from build123d import *

# Parameters (mm, degrees)
SKETCH046_R     = 1.5
PAD026_DEPTH    = 32
POCKET016_DEPTH = 21
SKETCH049_W     = 38.6999153105
SKETCH049_H     = 8
POCKET017_DEPTH = 50
PAD027_DEPTH    = 3
SKETCH050_W     = 42.8952211791
SKETCH050_H     = 8
POCKET018_DEPTH = 32
SKETCH051_R     = 23.5
PAD028_DEPTH    = 1


with BuildPart() as part:
    # Sketch046 → Pad026 (new body)
    with BuildSketch(Plane.XY):
        with BuildLine():
            Line((-21.3218441303, 2.7620577266), (-17, 2))
            Line((-17, 2), (-17, 1))
            Line((-17, 1), (-19, 1))
            Line((-19, 1), (-19, -1))
            Line((-19, -1), (-17, -1))
            Line((-17, -1), (-17, -2))
            Line((-19.3499576553, -2.4143609381), (-17, -2))
            ThreePointArc((-19.3499576553, -2.4143609381), (-18.5993421546, -5.8578555305), (-17.2411687539, -9.11))
            Line((17.2411687539, -9.11), (-17.2411687539, -9.11))
            ThreePointArc((17.2411687539, -9.11), (18.5993421546, -5.8578555305), (19.3499576553, -2.4143609381))
            Line((19.3499576553, -2.4143609381), (17, -2))
            Line((17, -2), (17, -1))
            Line((17, -1), (19, -1))
            Line((19, -1), (19, 1))
            Line((19, 1), (17, 1))
            Line((17, 1), (17, 2))
            Line((17, 2), (21.3218441303, 2.7620577266))
            ThreePointArc((13, -17.1245437895), (19.8334685845, -8.2996098649), (21.3218441303, 2.7620577266))
            Line((13, -17.1245437895), (10, -17.1245437895))
            Line((10, -17.1245437895), (10, -10.1245437895))
            Line((10, -10.1245437895), (-10, -10.1245437895))
            Line((-10, -10.1245437895), (-10, -17.1245437895))
            Line((-10, -17.1245437895), (-13, -17.1245437895))
            ThreePointArc((-21.3218441303, 2.7620577266), (-19.8334685845, -8.2996098649), (-13, -17.1245437895))
        make_face()
        with Locations((-12.5, -15)):
            Circle(SKETCH046_R, mode=Mode.SUBTRACT)
        with Locations((12.5, -15)):
            Circle(SKETCH046_R, mode=Mode.SUBTRACT)
    extrude(amount=PAD026_DEPTH)

    # Sketch047 (on Face28 of Pad026) → Pocket016 (cut)
    with BuildSketch(Plane.XY.offset(32)):
        with BuildLine():
            ThreePointArc((-18.9669083684, -10.1245437895), (-16.3621761284, -13.9473722379), (-13, -17.1245437895))
            Line((-13, -17.1245437895), (13, -17.1245437895))
            ThreePointArc((13, -17.1245437895), (16.3621761284, -13.9473722379), (18.9669083684, -10.1245437895))
            Line((-18.9669083684, -10.1245437895), (18.9669083684, -10.1245437895))
        make_face()
    extrude(amount=-POCKET016_DEPTH, mode=Mode.SUBTRACT)

    # Sketch049 (on Face5 of Pocket016) → Pocket017 (cut)
    with BuildSketch(Plane.XY.offset(32)):
        with Locations((0, 1.5856390619)):
            Rectangle(SKETCH049_W, SKETCH049_H)
    extrude(amount=-POCKET017_DEPTH, mode=Mode.SUBTRACT)

    # Sketch048 (on Face5 of Pocket016) → Pad027 (join)
    with BuildSketch(Plane.XY.offset(32)):
        with BuildLine():
            ThreePointArc((-21.4476105895, 1.5), (-21.02655084, -4.4871104034), (-18.9669083684, -10.1245437895))
            Line((-13, -10.1245437895), (-18.9669083684, -10.1245437895))
            Line((-6, -17.1245437895), (-13, -10.1245437895))
            Line((6, -17.1245437895), (-6, -17.1245437895))
            Line((6, -17.1245437895), (13, -10.1245437895))
            Line((13, -10.1245437895), (18.9669083684, -10.1245437895))
            ThreePointArc((18.9669083684, -10.1245437895), (21.02655084, -4.4871104034), (21.4476105895, 1.5))
            Line((-21.4476105895, 1.5), (21.4476105895, 1.5))
        make_face()
    extrude(amount=PAD027_DEPTH)

    # Sketch050 (on Face24 of Pad027) → Pocket018 (cut)
    with BuildSketch(Plane.XY.offset(32)):
        with Locations((0, 5.5)):
            Rectangle(SKETCH050_W, SKETCH050_H)
    extrude(amount=-POCKET018_DEPTH, mode=Mode.SUBTRACT)

    # Sketch051 (on Face27 of Pocket018) → Pad028 (join)
    with BuildSketch(Plane.XY.offset(35)):
        Circle(SKETCH051_R)
    extrude(amount=PAD028_DEPTH)


with BuildPart() as part_1:
    # Body018 placement: moved
    add(part.part.moved(Location((0, 0, 200))))


solid = part_1.part
Input: part model. Units: mm. Frame: model coordinates. A direction names the side the tool comes from. Coordinates: 2 decimals unless noted, no trailing zeros. Loops run counter-clockwise (first coordinate to the right, second up) from the corner with the lowest first, then second, coordinate; pieces in that order, holes last. Notation, with made-up numbers: (-13.5, 7.25) - (21.5, 7.25) arc R7 ccw to (21.5, 20.25) - close; hole circle Ø9 at (-35.5, 70.5). An arc over 180 degrees is marked (long way). Answer in a Markdown table with one row per item. Add a question column.
Item 1: Section query B-B on z = 209.5. Return the cut outline in (x, y).
Item 2: Section query A-A on y = -15. Return the cut outline in (x, z), then the cut area to 3 significant figures.
Item 3: Mould query, pull axis Y, two halves, no side actions, for faces 5 (the flat face through (0, 1.5, 233)), 6 (the cylindrical face through (-14, -15, 205)), 7 (the flat face through (13, -13, 211)). Classes: released by +Y, released by -Y, zero draft, split by the parting line, or undercut.
Item 4: Access query for faces 1 (the flat face through (-19.35, 0, 216)), 2 (the flat face through (0, -17.125, 233)), 3 (the cylindrical face through (11, -15, 205)), 4 (the flat face through (9.451, -13.674, 233.479)). Directions: +Z, -Z, +X, -X, +Y, -Y. A direction counts if a zero-diameter tool reaches every point of the face in a straight line with its end or side. Return the directions, or none.
Item 5: Section query C-C on z = 230.5. Return the cut outline in (x, y).
Item 6: Line query: line 1 along X through (y, z) = (-15, 202.75); line 2 along Y through (x, z) = (-12.5, 207.5); line 3 along Y through (x, z) = (-11, 216). Output: solid intervals per line, ascending. Write a range as [from, to].
Item 7: Section query D-D on x = 0. Return the cut outline in (y, z), then the cut area to 3 significant figures.
Item 8: Contact query for flat-ended pins moving along their axis: P1, Ø11.5, axis at x = 9, y = -3.5, coming from the -Z side; P2, Ø1.5, axis at y = -15.5, z = 211.5, coming from the +X side; P3, Ø5.5, axis at y = -15, z = 207.5, coming from the -X side; P4, Ø5, axis at x = 0.5, y = -17, coming from the -Z side. Output: stop coordinate, or through.
Recorded:
| question | item | result |
|---|---|---|
| 1 | outline | (-21.45, 1.5) arc R21.5 ccw to (-13, -17.12) - (-10, -17.12) - (-10, -10.12) - (10, -10.12) - (10, -17.12) - (13, -17.12) arc R21.5 ccw to (21.45, 1.5) - (19.35, 1.5) - (19.35, -2.41) arc R19.5 cw to (17.24, -9.11) - (-17.24, -9.11) arc R19.5 cw to (-19.35, -2.41) - (-19.35, 1.5) - close; hole circle Ø3 at (-12.5, -15); hole circle Ø3 at (12.5, -15) |
| 2 | outline | (-18.09, 235) - (-8.12, 235) - (-8.12, 232) - (8.12, 232) - (8.12, 235) - (18.09, 235) - (18.09, 236) - (-18.09, 236) - close; (-15.4, 200) - (-14, 200) - (-14, 211) - (-15.4, 211) - close; (-11, 200) - (-10, 200) - (-10, 211) - (-11, 211) - close; (10, 200) - (11, 200) - (11, 211) - (10, 211) - close; (14, 200) - (15.4, 200) - (15.4, 211) - (14, 211) - close |
| 2 | area | 138 mm^2 |
| 3 | face 5 | released by +Y |
| 3 | face 6 | undercut |
| 3 | face 7 | zero draft |
| 4 | face 1 | -Z, +Y |
| 4 | face 2 | -Z, +X, -X, -Y |
| 4 | face 3 | -Z |
| 4 | face 4 | +X, -Y |
| 5 | outline | (-21.45, 1.5) arc R21.5 ccw to (-18.97, -10.12) - (18.97, -10.12) arc R21.5 ccw to (21.45, 1.5) - (19.35, 1.5) - (19.35, -2.41) arc R19.5 cw to (17.24, -9.11) - (-17.24, -9.11) arc R19.5 cw to (-19.35, -2.41) - (-19.35, 1.5) - close |
| 6 | line 1 | [-15.4, -14], [-11, -10], [10, 11], [14, 15.4] |
| 6 | line 2 | [-17.12, -16.5], [-13.5, -9.11] |
| 6 | line 3 | [-10.12, -9.11] |
| 7 | outline | (-23.5, 235) - (-17.12, 235) - (-17.12, 232) - (-10.12, 232) - (-10.12, 200) - (-9.11, 200) - (-9.11, 232) - (1.5, 232) - (1.5, 235) - (23.5, 235) - (23.5, 236) - (-23.5, 236) - close |
| 7 | area | 135 mm^2 |
| 8 | P1 | z = 200 |
| 8 | P2 | x = 15.46 |
| 8 | P3 | x = -17.67 |
| 8 | P4 | z = 232 |
